Design review of the part built by this model. Coordinates are the model's own, in mm. A direction names the side the tool comes from. Give positions to 0.01 mm unless a question says otherwise; leave off trailing zeros. Order: outer loops, then holes, each group sorted by start corner. A loop starts at its lowest first (then second) coordinate and runs counter-clockwise, first axis right, second up.
```python
from build123d import *

# Parameters (mm, degrees)
SKETCH1_R          = 3.3274
EXTRUDE1_DEPTH     = 217.932
CUT_EXTRUDE1_DEPTH = 127


with BuildPart() as part:
    # Sketch1 → Extrude1 (new body)
    with BuildSketch(Plane.XY):
        with BuildLine():
            Line((-10.022898969, 12.91475973), (-5.252158105, 8.144007132))
            ThreePointArc((-5.252158105, 8.144007132), (-3.715177372, 7.117027388), (-1.902183975, 6.7564))
            Line((-1.902183975, 6.7564), (1.902183975, 6.7564))
            ThreePointArc((1.902183975, 6.7564), (3.715177372, 7.117027388), (5.252158105, 8.144007132))
            Line((5.252158105, 8.144007132), (10.022898969, 12.91475973))
            ThreePointArc((10.022898969, 12.91475973), (10.218362387, 13.207291992), (10.287, 13.552357131))
            Line((10.287, 13.552357131), (10.287, 14.0843))
            ThreePointArc((10.287, 14.0843), (10.022898185, 14.721898185), (9.3853, 14.986))
            Line((9.3853, 14.986), (5.617617549, 14.986))
            ThreePointArc((5.617617549, 14.986), (4.519044045, 15.441044045), (4.064, 16.539617549))
            Line((4.064, 16.539617549), (4.064, 17.496382451))
            ThreePointArc((4.064, 17.496382451), (4.519044045, 18.594955955), (5.617617549, 19.05))
            Line((5.617617549, 19.05), (7.974178704, 19.05))
            ThreePointArc((7.974178704, 19.05), (8.736178704, 18.288), (9.498178704, 19.05))
            Line((9.498178704, 19.05), (14.327719207, 19.05))
            ThreePointArc((14.327719207, 19.05), (15.087603123, 18.231251131), (15.847487039, 19.05))
            ThreePointArc((15.847487039, 19.05), (18.120176289, 18.120192083), (19.05, 15.847509295))
            ThreePointArc((19.05, 15.847509295), (18.231250992, 15.08762539), (19.05, 14.327741484))
            Line((19.05, 14.327741484), (19.05, 9.496091471))
            ThreePointArc((19.05, 9.496091471), (18.231250992, 8.736207565), (19.05, 7.97632366))
            Line((19.05, 7.97632366), (19.05, 5.617617549))
            ThreePointArc((19.05, 5.617617549), (18.594955955, 4.519044045), (17.496382451, 4.064))
            Line((17.496382451, 4.064), (16.539617549, 4.064))
            ThreePointArc((16.539617549, 4.064), (15.441044045, 4.519044045), (14.986, 5.617617549))
            Line((14.986, 5.617617549), (14.986, 9.385342516))
            ThreePointArc((14.986, 9.385342516), (14.721898185, 10.022940701), (14.0843, 10.287042516))
            Line((14.0843, 10.287042516), (13.516042086, 10.287042516))
            ThreePointArc((13.516042086, 10.287042516), (13.170975923, 10.218404478), (12.878443117, 10.022939917))
            Line((12.878443117, 10.022939917), (8.14758008, 5.292065243))
            ThreePointArc((8.14758008, 5.292065243), (7.117955879, 3.751120653), (6.7564, 1.933453584))
            Line((6.7564, 1.933453584), (6.7564, -1.933453584))
            ThreePointArc((6.7564, -1.933453584), (7.117955879, -3.751120653), (8.14758008, -5.292065243))
            Line((8.14758008, -5.292065243), (12.878443117, -10.022939917))
            ThreePointArc((12.878443117, -10.022939917), (13.170975923, -10.218404478), (13.516042086, -10.287042516))
            Line((13.516042086, -10.287042516), (14.0843, -10.287042516))
            ThreePointArc((14.0843, -10.287042516), (14.721898185, -10.022940701), (14.986, -9.385342516))
            Line((14.986, -9.385342516), (14.986, -5.617617549))
            ThreePointArc((14.986, -5.617617549), (15.441044045, -4.519044045), (16.539617549, -4.064))
            Line((16.539617549, -4.064), (17.496382451, -4.064))
            ThreePointArc((17.496382451, -4.064), (18.594955955, -4.519044045), (19.05, -5.617617549))
            Line((19.05, -5.617617549), (19.05, -7.976318491))
            ThreePointArc((19.05, -7.976318491), (18.231250992, -8.736202396), (19.05, -9.496086302))
            Line((19.05, -9.496086302), (19.05, -14.32774291))
            ThreePointArc((19.05, -14.32774291), (18.231250992, -15.087626816), (19.05, -15.847510721))
            ThreePointArc((19.05, -15.847510721), (18.120175716, -18.120192644), (15.847486868, -19.05))
            ThreePointArc((15.847486868, -19.05), (15.087602952, -18.231251131), (14.327719036, -19.05))
            Line((14.327719036, -19.05), (9.496062448, -19.05))
            ThreePointArc((9.496062448, -19.05), (8.736178532, -18.231251131), (7.976294616, -19.05))
            Line((7.976294616, -19.05), (5.617617549, -19.05))
            ThreePointArc((5.617617549, -19.05), (4.519044045, -18.594955955), (4.064, -17.496382451))
            Line((4.064, -17.496382451), (4.064, -16.539617549))
            ThreePointArc((4.064, -16.539617549), (4.519044045, -15.441044045), (5.617617549, -14.986))
            Line((5.617617549, -14.986), (9.3853, -14.986))
            ThreePointArc((9.3853, -14.986), (10.022898185, -14.721898185), (10.287, -14.0843))
            Line((10.287, -14.0843), (10.287, -13.552357131))
            ThreePointArc((10.287, -13.552357131), (10.218362387, -13.207291992), (10.022898969, -12.91475973))
            Line((10.022898969, -12.91475973), (5.252158105, -8.144007132))
            ThreePointArc((5.252158105, -8.144007132), (3.715177372, -7.117027388), (1.902183975, -6.7564))
            Line((1.902183975, -6.7564), (-1.902183975, -6.7564))
            ThreePointArc((-1.902183975, -6.7564), (-3.715177372, -7.117027388), (-5.252158105, -8.144007132))
            Line((-5.252158105, -8.144007132), (-10.022898969, -12.91475973))
            ThreePointArc((-10.022898969, -12.91475973), (-10.218362387, -13.207291992), (-10.287, -13.552357131))
            Line((-10.287, -13.552357131), (-10.287, -14.0843))
            ThreePointArc((-10.287, -14.0843), (-10.022898185, -14.721898185), (-9.3853, -14.986))
            Line((-9.3853, -14.986), (-5.617617549, -14.986))
            ThreePointArc((-5.617617549, -14.986), (-4.519044045, -15.441044045), (-4.064, -16.539617549))
            Line((-4.064, -16.539617549), (-4.064, -17.496382451))
            ThreePointArc((-4.064, -17.496382451), (-4.519044045, -18.594955955), (-5.617617549, -19.05))
            Line((-5.617617549, -19.05), (-7.976294616, -19.05))
            ThreePointArc((-7.976294616, -19.05), (-8.736178532, -18.231251131), (-9.496062448, -19.05))
            Line((-9.496062448, -19.05), (-14.327719036, -19.05))
            ThreePointArc((-14.327719036, -19.05), (-15.087602952, -18.231251131), (-15.847486868, -19.05))
            ThreePointArc((-15.847486868, -19.05), (-18.120175716, -18.120192644), (-19.05, -15.847510721))
            ThreePointArc((-19.05, -15.847510721), (-18.231250992, -15.087626816), (-19.05, -14.32774291))
            Line((-19.05, -14.32774291), (-19.05, -9.496086302))
            ThreePointArc((-19.05, -9.496086302), (-18.231250992, -8.736202396), (-19.05, -7.976318491))
            Line((-19.05, -7.976318491), (-19.05, -5.617617549))
            ThreePointArc((-19.05, -5.617617549), (-18.594955955, -4.519044045), (-17.496382451, -4.064))
            Line((-17.496382451, -4.064), (-16.539617549, -4.064))
            ThreePointArc((-16.539617549, -4.064), (-15.441044045, -4.519044045), (-14.986, -5.617617549))
            Line((-14.986, -5.617617549), (-14.986, -9.385342516))
            ThreePointArc((-14.986, -9.385342516), (-14.721898185, -10.022940701), (-14.0843, -10.287042516))
            Line((-14.0843, -10.287042516), (-13.516042086, -10.287042516))
            ThreePointArc((-13.516042086, -10.287042516), (-13.170975923, -10.218404478), (-12.878443117, -10.022939917))
            Line((-12.878443117, -10.022939917), (-8.14758008, -5.292065243))
            ThreePointArc((-8.14758008, -5.292065243), (-7.117955879, -3.751120653), (-6.7564, -1.933453584))
            Line((-6.7564, -1.933453584), (-6.7564, 1.933453584))
            ThreePointArc((-6.7564, 1.933453584), (-7.117955879, 3.751120653), (-8.14758008, 5.292065243))
            Line((-8.14758008, 5.292065243), (-12.878443117, 10.022939917))
            ThreePointArc((-12.878443117, 10.022939917), (-13.170975923, 10.218404478), (-13.516042086, 10.287042516))
            Line((-13.516042086, 10.287042516), (-14.0843, 10.287042516))
            ThreePointArc((-14.0843, 10.287042516), (-14.721898185, 10.022940701), (-14.986, 9.385342516))
            Line((-14.986, 9.385342516), (-14.986, 5.617617549))
            ThreePointArc((-14.986, 5.617617549), (-15.441044045, 4.519044045), (-16.539617549, 4.064))
            Line((-16.539617549, 4.064), (-17.496382451, 4.064))
            ThreePointArc((-17.496382451, 4.064), (-18.594955955, 4.519044045), (-19.05, 5.617617549))
            Line((-19.05, 5.617617549), (-19.05, 7.97632366))
            ThreePointArc((-19.05, 7.97632366), (-18.231250992, 8.736207565), (-19.05, 9.496091471))
            Line((-19.05, 9.496091471), (-19.05, 14.327741484))
            ThreePointArc((-19.05, 14.327741484), (-18.231250992, 15.08762539), (-19.05, 15.847509295))
            ThreePointArc((-19.05, 15.847509295), (-18.120176289, 18.120192083), (-15.847487039, 19.05))
            ThreePointArc((-15.847487039, 19.05), (-15.087603123, 18.231251131), (-14.327719207, 19.05))
            Line((-14.327719207, 19.05), (-9.498178704, 19.05))
            ThreePointArc((-9.498178704, 19.05), (-8.736178704, 18.288), (-7.974178704, 19.05))
            Line((-7.974178704, 19.05), (-5.617617549, 19.05))
            ThreePointArc((-5.617617549, 19.05), (-4.519044045, 18.594955955), (-4.064, 17.496382451))
            Line((-4.064, 17.496382451), (-4.064, 16.539617549))
            ThreePointArc((-4.064, 16.539617549), (-4.519044045, 15.441044045), (-5.617617549, 14.986))
            Line((-5.617617549, 14.986), (-9.3853, 14.986))
            ThreePointArc((-9.3853, 14.986), (-10.022898185, 14.721898185), (-10.287, 14.0843))
            Line((-10.287, 14.0843), (-10.287, 13.552357131))
            ThreePointArc((-10.287, 13.552357131), (-10.218362387, 13.207291992), (-10.022898969, 12.91475973))
        make_face()
        Circle(SKETCH1_R, mode=Mode.SUBTRACT)
    extrude(amount=-EXTRUDE1_DEPTH)

    # Sketch2 → Cut-Extrude1 (cut)
    with BuildSketch(Plane(origin=(0, 19.05, 0), x_dir=(1, 0, 0), z_dir=(0, 1, 0))):
        Polygon((19.05, 0), (-19.05, 2.664211535), (-19.05, 0), align=None)
    extrude(amount=-CUT_EXTRUDE1_DEPTH, mode=Mode.SUBTRACT)


solid = part.part
```
1. Draft analysis for pull direction X (two halves, no side actions). For faces 1 (the face through (-12, 19.05, -108)), 2 (the face through (-8, -14.986, -108)), 3 (the face through (19.05, -12, -107)), state which applies: pulls with the +X half, pulls with the -X half, needs draft (parallel to the pull), parting line crosses it, or undercut.
Recorded:
face 1: needs draft
face 2: undercut
face 3: pulls with the +X half
2. Machinability: for faces 4 (the face through (12, -19.05, -108)), 5 (the face through (5, 0, -217.932)), 6 (the face through (-14.986, 8, -109)), 7 (the face through (0, -6.756, -108)), 8 (the face through (6.756, 0, -108)), which of the approach directions +Z, -Z, +X, -X, +Y, -Y give a long, thin tool a straight path to every point of the face, cutting with its end or side? Answer none if there is none.
Recorded:
face 4: +Z, -Z, +X, -X, -Y
face 5: -Z, +X, -X, +Y, -Y
face 6: +Z, -Z
face 7: +Z, -Z, -Y
face 8: +Z, -Z, +X
3. For pin 1 (4 mm diameter, centred on y = -2.5, z = -193.5, fed in from +X); pin 2 (2 mm diameter, centred on x = 13.5, y = -10, fed in from -Z); pin 3 (1.5 mm diameter, centred on x = 1, z = -80.5, fed in from +Y); pin 4 (1.1 mm diameter, centred on x = -17, z = -105, fed in from +Y), all flat-tipped, find the tip position at first contact; note any pin that passes through.
Recorded:
pin 1: stops at x = 18.58
pin 2: stops at z = -217.93
pin 3: stops at y = 6.76
pin 4: stops at y = 19
4. For line 1 along Y through (x, z) = (0, -166); line 2 along X through (y, z) = (-5, -28); line 3 along X through (y, z) = (6.5, -165), list the stretches that pass through material, from the lowest coordinate up.
Recorded:
line 1: y = -6.76 to -3.33, 3.33 to 6.76
line 2: x = -18.92 to -15.11, -7.88 to 7.88, 15.11 to 18.92
line 3: x = -19.05 to -14.99, -9.36 to 9.36, 14.99 to 19.05
5. Take a section at B-B (x = 0). State the section outline as (y, z) points.
Recorded:
outline: (-6.76, -217.93) - (-3.33, -217.93) - (-3.33, -1.33) - (-6.76, -1.33) - close; (3.33, -217.93) - (6.76, -217.93) - (6.76, -1.33) - (3.33, -1.33) - close
6. Take a section at A-A (y = 0). State the section outline as (x, z) points.
Recorded:
outline: (-6.76, -217.93) - (-3.33, -217.93) - (-3.33, -1.56) - (-6.76, -1.8) - close; (3.33, -217.93) - (6.76, -217.93) - (6.76, -0.86) - (3.33, -1.1) - close
